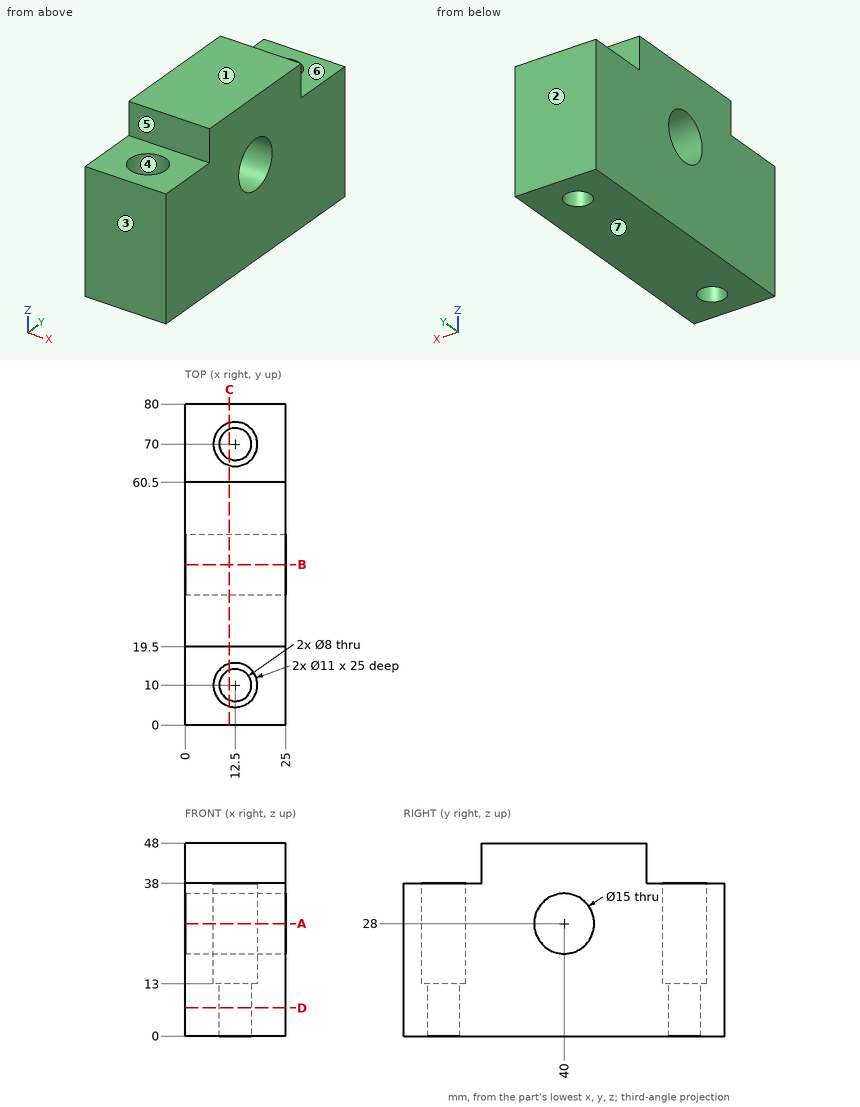
Source: three-view drawing plus pictorial views. Frame: mm from the lowest corner of the part. A direction names the side the tool comes from. Give positions to 0.01 mm unless a question says otherwise; leave off trailing zeros. Order: outer loops, then holes, each group sorted by start corner. A loop starts at its lowest first (then second) coordinate and runs counter-clockwise, first axis right, second up. Notation, with made-up numbers: M 33,74.25 L 75,74.25 A10 cw 75,88.25 Z; hole C -39,82.5 d10. An arc over 180 degrees is marked long. Return JSON: item names as keys, results as strings.
1) Contact query for flat-ended pins moving along their axis: pin 1 (12 mm diameter, centred on x = 15, y = 52, fed in from -Z); pin 2 (12 mm diameter, centred on x = 13.5, y = 9.5, fed in from +Z); pin 3 (11 mm diameter, centred on x = 13.5, z = 45, fed in from +Y); pin 4 (10 mm diameter, centred on x = 12.5, y = 10, fed in from +Z). Output: stop coordinate, or through.
Taken from the geometry:
{"pin 1": "stops at z = 0", "pin 2": "stops at z = 38", "pin 3": "stops at y = 60.5", "pin 4": "stops at z = 13"}
2) Section query B-B on y = 40. Output: boundary loops of the cut face in (x, z), and give its area (3 significant figures).
Taken from the geometry:
{"outline": "M 0,0 L 25,0 L 25,20.5 L 0,20.5 Z; M 0,35.5 L 25,35.5 L 25,48 L 0,48 Z", "area": "825 mm2"}
3) Section query C-C on x = 11. Output: boundary loops of the cut face in (y, z).
Taken from the geometry:
{"outline": "M 0,0 L 6.29,0 L 6.29,13 L 4.71,13 L 4.71,38 L 0,38 Z; M 13.71,0 L 66.29,0 L 66.29,13 L 64.71,13 L 64.71,38 L 60.5,38 L 60.5,48 L 19.5,48 L 19.5,38 L 15.29,38 L 15.29,13 L 13.71,13 Z; M 73.71,0 L 80,0 L 80,38 L 75.29,38 L 75.29,13 L 73.71,13 Z; hole C 40,28 d15"}
4) Access query for the marked faces 5, 6 and 7. Directions: +Z, -Z, +X, -X, +Y, -Y. A direction counts if a zero-diameter tool reaches every point of the face in a straight line with its end or side. Return the directions, or none.
Taken from the geometry:
{"face 5": "+Z, +X, -X, -Y", "face 6": "+Z, +X, -X, +Y", "face 7": "-Z, +X, -X, +Y, -Y"}
5) Line query: L1, parallel to Y at x = 9.25, z = 25; L2, parallel to Y at x = 12.5, z = 22.5; L3, parallel to Y at x = 15.25, z = 2. Output: solid intervals per line, ascending. Write a range as [from, to].
Taken from the geometry:
{"L1": "y = [0, 5.56], [14.44, 33.13], [46.87, 65.56], [74.44, 80]", "L2": "y = [0, 4.5], [15.5, 34.9], [45.1, 64.5], [75.5, 80]", "L3": "y = [0, 7.1], [12.9, 67.1], [72.9, 80]"}
6) Mould query, pull axis Y, two halves, no side actions, for the marked faces 1, 2, 3 and 4. Classes: released by +Y, released by -Y, zero draft, split by the parting line, or undercut.
Taken from the geometry:
{"face 1": "zero draft", "face 2": "released by +Y", "face 3": "released by -Y", "face 4": "undercut"}
7) Section query D-D on z = 7. Output: boundary loops of the cut face in (x, y), and give its area (3 significant figures).
Taken from the geometry:
{"outline": "M 0,0 L 25,0 L 25,80 L 0,80 Z; hole C 12.5,10 d8; hole C 12.5,70 d8", "area": "1,900 mm2"}
8) Section query A-A on z = 28. Output: boundary loops of the cut face in (x, y).
Taken from the geometry:
{"outline": "M 0,0 L 25,0 L 25,32.5 L 0,32.5 Z; M 0,47.5 L 25,47.5 L 25,80 L 0,80 Z; hole C 12.5,10 d11; hole C 12.5,70 d11"}
